Autodesk Inventor part; units mm, degrees
ref_plane "YZ Plane" through (0, 0, 0) normal (1, 0, 0) x (0, 1, 0)
ref_plane "XZ Plane" through (0, 0, 0) normal (0, 1, 0) x (-1, 0, 0)
ref_plane "XY Plane" through (0, 0, 0) normal (0, 0, 1) x (1, 0, 0)
sketch "Sketch1" plane through (0, 0, 0) normal (0, 0, 1) x (1, 0, 0)
  line L0 (0, 43) -> (77, 43)
  line L1 (77, 43) -> (77, 0)
  line L2 (77, 0) -> (0, 0)
  line L3 (0, 0) -> (0, 43)
  point P0 (74.8142, 2.33)
  point P1 (74.8142, 51.9717)
  dimension "d0" = 77
  dimension "d1" = 43
extrude "Extrusion1" add sketch "Sketch1" along normal blind 6
sketch "Sketch2" plane through (0, 0, 6) normal (0, 0, 1) x (1, 0, 0)
  point P0 (0, 0)
sketch "Sketch3" plane through (0, 0, 6) normal (0, 0, 1) x (1, 0, 0)
  line L0 (9, 43) -> (70, 43)
  line L1 (70, 43) -> (70, 0)
  line L2 (70, 0) -> (9, 0)
  line L3 (9, 0) -> (9, 43)
  line L4 (77, 0) -> (77, 43)
  line L5 (0, 0) -> (77, 0)
  line L6 (77, 43) -> (0, 43)
  point P0 (75, 41)
  point P1 (75, 2)
  dimension "d4" = 61
  dimension "d5" = 7
  dimension "d6" = 2
  dimension "d7" = 2
  dimension "d8" = 2
extrude "Extrusion2" add sketch "Sketch3" along normal blind 6 contours L0 L1 L2 L3
sketch "Sketch4" plane through (0, 0, 6) normal (0, 0, 1) x (1, 0, 0)
  line L0 (77, 43) -> (70, 43)
  line L1 (70, 0) -> (77, 0)
  line L2 (77, 0) -> (77, 43)
  point P0 (0, 0)
  point P1 (75, 2)
  point P2 (75, 41)
  dimension "d11" = 2
  dimension "d12" = 2
  dimension "d13" = 2
hole "Hole1" at (75, 2, 6) at (75, 41, 6) direction (0, 0, -1) diameter 3 end through all
sketch "Sketch5" plane through (0, 0, 6) normal (0, 0, 1) x (1, 0, 0)
  line L0 (9, 43) -> (0, 43)
  line L1 (0, 0) -> (9, 0)
  line L2 (0, 43) -> (0, 0)
  point P0 (6.5, 2)
  point P1 (6.5, 41)
  dimension "d21" = 2
  dimension "d22" = 2
  dimension "d23" = 6.5
hole "Hole2" at (6.5, 41, 6) at (6.5, 2, 6) direction (0, 0, -1) diameter 3 end through all
properties part number "Pantalla"
Input: part model. Units: mm. Frame: model coordinates. A direction names the side the tool comes from. Give positions to 0.01 mm unless a question says otherwise; leave off trailing zeros. Write each loop counter-clockwise with the first axis right and the second up, starting at its lowest first coordinate (ties: lowest second). Pieces come first, ordered by that corner, then holes. Notation, with made-up numbers: (81.25, 28.5) - (127.25, 28.5) arc R19 ccw to (127.25, 42.5) - close; hole circle Ø6 at (51, 7). An arc over 180 degrees is marked (long way). Write item = value, one per line. Start each with the question number.
1. First-contact query: pin 1 Ø2.5 at (x, y) = (6.5, 2) entering from -Z; pin 2 Ø6.5 at (y, z) = (18.5, 8) entering from +X; pin 3 Ø6.5 at (y, z) = (28.5, 10) entering from -X; pin 4 Ø7.5 at (x, y) = (74.5, 14.5) entering from +Z. Flat tips, straight axial feed; report the tip coordinate or a pass-through.
2. Mould query, pull axis Y, two halves, no side actions, for faces 4 (the cylindrical face through (7.83, 1.31, 2.96)), 5 (the flat face through (9, 21, 9)), 6 (the cylindrical face through (6.43, 42.5, 2.96)), 7 (the flat face through (38, 43, 6)). Classes: released by +Y, released by -Y, zero draft, split by the parting line, or undercut.
3. Section query C-C, the plane y = 36. Output: boundary loops of the cut face in (x, z), then the cut area to 3 significant figures.
4. Section query A-A, the plane x = 6.5. Output: boundary loops of the cut face in (y, z).
5. Section query B-B, the plane y = 41. Output: boundary loops of the cut face in (x, z).
6. Section query D-D, the plane z = 7.5. Output: boundary loops of the cut face in (x, y).
7. Access query for faces 1 (the flat face through (4, 22, 6)), 2 (the flat face through (73, 22, 6)), 3 (the cylindrical face through (73.99, 42.11, 2.96)). Directions: +Z, -Z, +X, -X, +Y, -Y. A direction counts if a zero-diameter tool reaches every point of the face in a straight line with its end or side. Return the directions, or none.
8. Ray query, L1, parallel to X at y = 41, z = 1.45; L2, parallel to Y at x = 75, z = 4.6; L3, parallel to X at y = 3, z = 11. Return the intervals inside material, ascending.
Check sheet entries:
q1.pin_1 = through
q1.pin_2 = 77
q1.pin_3 = 9
q1.pin_4 = 6
q2.face_4 = undercut
q2.face_5 = zero draft
q2.face_6 = undercut
q2.face_7 = released by +Y
q3.outline = (0, 0) - (77, 0) - (77, 6) - (70, 6) - (70, 12) - (9, 12) - (9, 6) - (0, 6) - close
q3.area = 828 mm2
q4.outline = (0, 0) - (0.5, 0) - (0.5, 6) - (0, 6) - close; (3.5, 0) - (39.5, 0) - (39.5, 6) - (3.5, 6) - close; (42.5, 0) - (43, 0) - (43, 6) - (42.5, 6) - close
q5.outline = (0, 0) - (5, 0) - (5, 6) - (0, 6) - close; (8, 0) - (73.5, 0) - (73.5, 6) - (70, 6) - (70, 12) - (9, 12) - (9, 6) - (8, 6) - close; (76.5, 0) - (77, 0) - (77, 6) - (76.5, 6) - close
q6.outline = (9, 0) - (70, 0) - (70, 43) - (9, 43) - close
q7.face_1 = +Z, -X, +Y, -Y
q7.face_2 = +Z, +X, +Y, -Y
q7.face_3 = +Z, -Z
q8.L1 = 0 to 5, 8 to 73.5, 76.5 to 77
q8.L2 = 0 to 0.5, 3.5 to 39.5, 42.5 to 43
q8.L3 = 9 to 70
